Part model, mm, in its own coordinate system. Round coordinates to 2 decimals unless told otherwise and drop trailing zeros. Loops run counter-clockwise (first coordinate to the right, second up) from the corner with the lowest first, then second, coordinate; pieces in that order, holes last.
1) Band-saw the part on B-B, the plane x = 15. Write the cut outline in (y, z).
2) Mould opens along Y. For faces 1 (the flat face through (44, 2, 5)), 2 (the cylindrical face through (63.513, 0.195, 4.493)) say: +Y half, -Y half, draft (parallel to the pull), parting line (faces both ways), or undercut.
3) Band-saw the part on A-A, the plane y = 2.25. Write the cut outline in (x, z), then the cut area to 3 significant figures.
4) Drop a flat-ended pin along its axis: P1, Ø3.5, axis at x = 85, y = 0, coming from the -Z side. Give the stop position or say it passes through.
5) Probe line 1 (Y direction, x = 79.5, z = 3.5); line 2 (Y direction, x = 15, z = -4.4). List the from-to ranges inside material, lowest first.
Autodesk Inventor part; units mm, degrees
ref_plane "YZ Plane" through (0, 0, 0) normal (1, 0, 0) x (0, 1, 0)
ref_plane "XZ Plane" through (0, 0, 0) normal (0, 1, 0) x (-1, 0, 0)
ref_plane "XY Plane" through (0, 0, 0) normal (0, 0, 1) x (1, 0, 0)
sketch "Sketch1" plane through (0, 0, 0) normal (1, 0, 0) x (0, 1, 0)
  line L0 (-5, -5) -> (5, -5)
  line L1 (5, -5) -> (5, 5)
  line L2 (5, 5) -> (-5, 5)
  line L3 (-5, 5) -> (-5, -5)
  line L4 (-5, -5) -> (5, 5) construction
  line L5 (5, -5) -> (-5, 5) construction
  line L6 (-4, -4) -> (4, -4)
  line L7 (4, -4) -> (4, 4)
  line L8 (4, 4) -> (-4, 4)
  line L9 (-4, 4) -> (-4, -4)
  line L10 (-4, -4) -> (4, 4) construction
  line L11 (4, -4) -> (-4, 4) construction
  point P0 (0, 0)
  dimension "d0" = 10
  dimension "d1" = 10
  dimension "d2" = 8
  dimension "d3" = 8
extrude "Extrusion1" add sketch "Sketch1" along normal blind 90
sketch "Sketch2" plane through (0, -5, 5) normal (0, 0, 1) x (1, 0, 0)
  line L0 (90, 10) -> (90, 0)
  line L1 (0, 10) -> (0, 0)
  line L2 (5, 5) -> (25.8215, 5)
  point P0 (0, 5)
  point P1 (15, 5)
  point P2 (15, 5)
  point P3 (25, 5)
  point P4 (25, 5)
  point P5 (35, 5)
  point P6 (35, 5)
  point P7 (45, 5)
  point P8 (45, 5)
  point P9 (55, 5)
  point P10 (55, 5)
  point P11 (65, 5)
  point P12 (65, 5)
  point P13 (75, 5)
  point P14 (75, 5)
  point P15 (85, 5)
  dimension "d7" = 5
  dimension "d15" = 10
  dimension "d18" = 10
hole "Hole1" at (5, 0, 5) at (15, 0, 5) at (25, 0, 5) at (35, 0, 5) at (45, 0, 5) at (55, 0, 5) at (65, 0, 5) at (75, 0, 5) at (85, 0, 5) direction (0, 0, -1) diameter 3 depth 80.45
sketch "Sketch3" plane through (0, 5, 5) normal (0, 1, 0) x (1, 0, 0)
  line L0 (0, 10) -> (0, 0)
  line L1 (0, 5) -> (10, 5)
  point P0 (20, 5)
  point P1 (20, 5)
  point P2 (30, 5)
  point P3 (30, 5)
  point P4 (40, 5)
  point P5 (40, 5)
  point P6 (50, 5)
  point P7 (50, 5)
  point P8 (60, 5)
  point P9 (60, 5)
  point P10 (70, 5)
  point P11 (70, 5)
  point P12 (80, 5)
  dimension "d23" = 10
  dimension "d24" = 10
  dimension "d27" = 10
hole "Hole2" at (10, 5, 0) at (20, 5, 0) at (30, 5, 0) at (40, 5, 0) at (50, 5, 0) at (60, 5, 0) at (70, 5, 0) at (80, 5, 0) direction (0, -1, 0) diameter 3 depth 80.45
sketch "Sketch4" plane through (0, 5, 5) normal (0, 1, 0) x (1, 0, 0)
  circle A0 centre (10, 5) radius 1.5
  point P0 (0, 5)
  point P1 (7.5, 5)
  dimension "d39" = 2.5
hole "Hole3" at (7.5, 5, 0) direction (0, -1, 0) diameter 3 depth 80.45
properties part number "10x10x60" material "アルミニウム 6061"
Reported:
1. outline: (-5, -5) - (-1.5, -5) - (-1.5, -4) - (-4, -4) - (-4, 4) - (-1.5, 4) - (-1.5, 5) - (-5, 5) - close; (1.5, -5) - (5, -5) - (5, 5) - (1.5, 5) - (1.5, 4) - (4, 4) - (4, -4) - (1.5, -4) - close
2. face 1: draft
2. face 2: undercut
3. outline: (0, -5) - (90, -5) - (90, -4) - (0, -4) - close; (0, 4) - (90, 4) - (90, 5) - (0, 5) - close
3. area: 180 mm2
4. P1: stops at z = -5
5. line 1: y = -5 to -4, 4 to 5
5. line 2: y = -5 to -1.5, 1.5 to 5
